Geometry check sheet. Reference: the model listing, model coordinates, mm. Face numbers are marked on the shaded views. A direction names the side the tool comes from. Coordinates: 2 decimals unless noted, no trailing zeros. Write each loop counter-clockwise with the first axis right and the second up, starting at its lowest first coordinate (ties: lowest second). Pieces come first, ordered by that corner, then holes.
from build123d import *

# Parameters (mm, degrees)
T_LE_DE_BASE_PLI_E1_DEPTH = 25
TROU_TARAUD_M31_D         = 2.5
D_GAGEMENT_M41_D          = 4.5


# Sheet-metal steps are written as plain solids
with BuildPart() as part:
    # Esquisse1 → Tôle de base pliée1 (new body)
    with BuildSketch(Plane(origin=(0, 0, 0), x_dir=(0, 0, -1), z_dir=(1, 0, 0))):
        with BuildLine():
            Line((0, 12.75), (0, 4))
            ThreePointArc((0, 4), (-1.171572875, 1.171572875), (-4, 0))
            Line((-4, 0), (-29, 0))
            Line((-29, 0), (-29, 3))
            Line((-29, 3), (-4, 3))
            ThreePointArc((-4, 3), (-3.292893219, 3.292893219), (-3, 4))
            Line((-3, 4), (-3, 12.75))
            Line((-3, 12.75), (0, 12.75))
        make_face()
    extrude(amount=T_LE_DE_BASE_PLI_E1_DEPTH)

    # Trou taraudé M31 (through all)
    with Locations(Plane(origin=(0, 3, 0), x_dir=(1, 0, 0), z_dir=(0, 1, 0))):
        with Locations((4.5, -24.5), (4.5, -8.5), (20.5, -8.5), (20.5, -24.5)):
            Hole(TROU_TARAUD_M31_D / 2)

    # Dégagement M41 (through all)
    with Locations(Plane.XY.offset(3)):
        with Locations((12.5, 8.2)):
            Hole(D_GAGEMENT_M41_D / 2)


solid = part.part
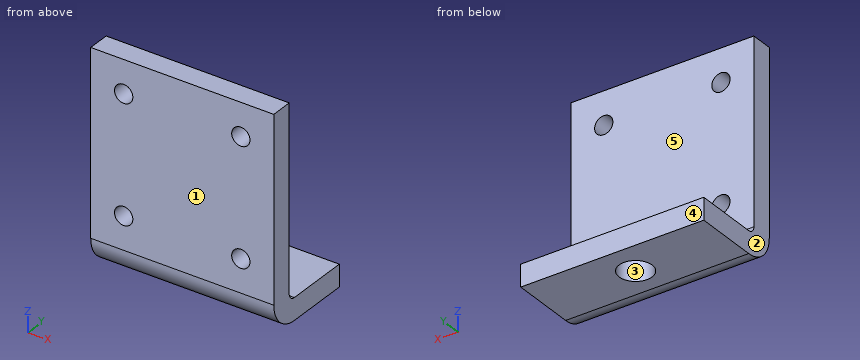
1. Sectioned sample at B-B, the plane z = 24.5. Record the boundary of the cut face in (x, y), and give its area (3 significant figures).
Computed values:
outline: (0, 0) - (3.25, 0) - (3.25, 3) - (0, 3) - close; (5.75, 0) - (19.25, 0) - (19.25, 3) - (5.75, 3) - close; (21.75, 0) - (25, 0) - (25, 3) - (21.75, 3) - close
area: 60.0 mm2
2. Sectioned sample at C-C, the plane x = 12.5. Record the boundary of the cut face in (y, z), and give its area (3 significant figures).
Computed values:
outline: (0, 4) arc R4 ccw to (4, 0) - (5.95, 0) - (5.95, 3) - (4, 3) arc R1 cw to (3, 4) - (3, 29) - (0, 29) - close; (10.45, 0) - (12.75, 0) - (12.75, 3) - (10.45, 3) - close
area: 99.5 mm2
3. Thickness scan on line 1 along X through (y, z) = (1.1, 8.5); line 2 along Z through (x, y) = (20.5, 2.2); line 3 along Y through (x, z) = (11, 25.5). Record the ranges inside material, lowest first.
Computed values:
line 1: x = 0 to 3.25, 5.75 to 19.25, 21.75 to 25
line 2: z = 0.43 to 7.25, 9.75 to 23.25, 25.75 to 29
line 3: y = 0 to 3
4. Draft check along Y on the marked faces 1, 2 and 3. Enter one of: released by +Y, released by -Y, zero draft, split by the parting line, or undercut.
Computed values:
face 1: released by -Y
face 2: zero draft
face 3: undercut
5. Sectioned sample at D-D, the plane x = 17.5. Record the boundary of the cut face in (y, z), and give its area (3 significant figures).
Computed values:
outline: (0, 4) arc R4 ccw to (4, 0) - (12.75, 0) - (12.75, 3) - (4, 3) arc R1 cw to (3, 4) - (3, 29) - (0, 29) - close
area: 113 mm2
6. Gauge pin test, flat ends, axial feed: pin 1 Ø4.5 at (x, y) = (17.5, 10.5) entering from +Z; pin 2 Ø2 at (x, z) = (4.5, 24.5) entering from -Y; pin 3 Ø12 at (x, z) = (22, 11) entering from +Y. Record the tip position at first contact, or that the pin passes through.
Computed values:
pin 1: stops at z = 3
pin 2: passes through
pin 3: stops at y = 3
7. Sectioned sample at A-A, the plane y = 8.2. Record the boundary of the cut face in (x, z), and give its area (3 significant figures).
Computed values:
outline: (0, 0) - (10.25, 0) - (10.25, 3) - (0, 3) - close; (14.75, 0) - (25, 0) - (25, 3) - (14.75, 3) - close
area: 61.5 mm2
8. Access from +Z, -Z, +X, -X, +Y, -Y to the whole of each face (thin tool, end or side, straight path). Record for the marked faces 4 and 5.
Computed values:
face 4: +Z, -Z, +X, -X, +Y
face 5: +Z, +X, -X, +Y
